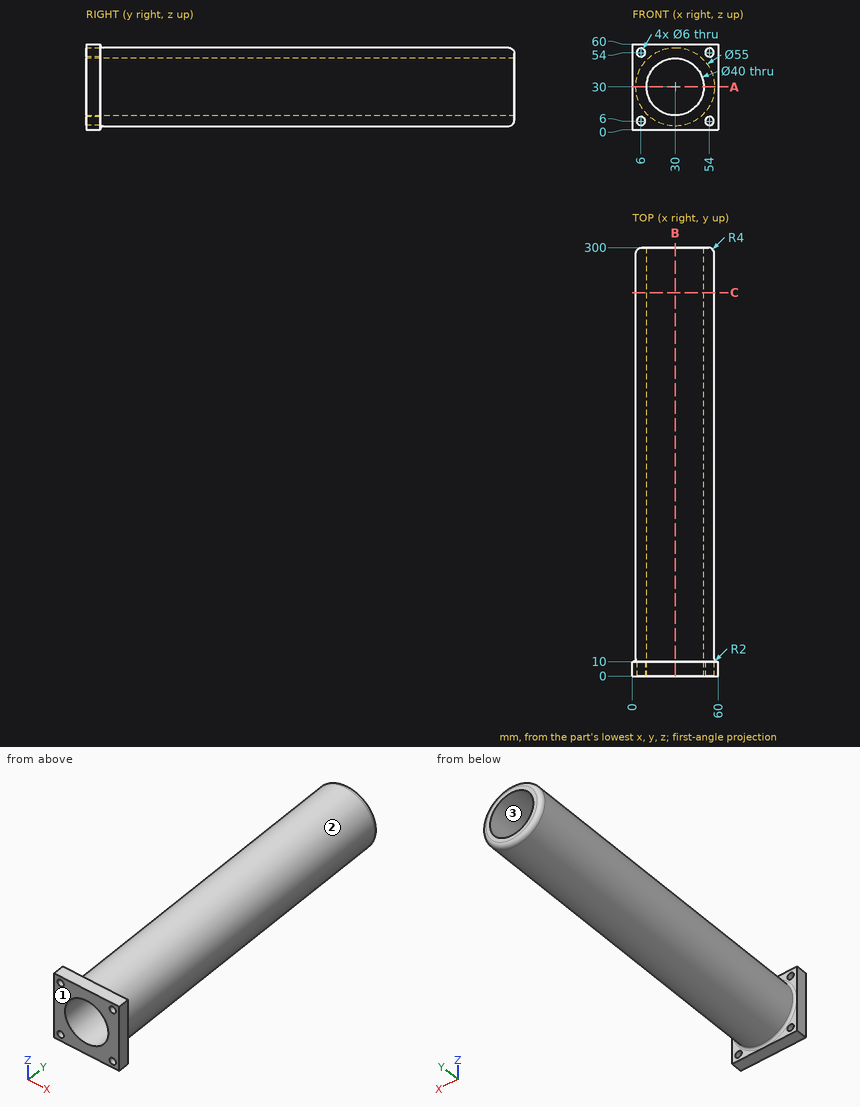
Design review of the part shown in the three views and the two pictorial views. Dimensions are in mm from the part's minimum x, y and z. Give positions to 0.01 mm unless a question says otherwise; leave off trailing zeros. Loops run counter-clockwise (first coordinate to the right, second up) from the corner with the lowest first, then second, coordinate; pieces in that order, holes last. Notation, with made-up numbers: (20, 55.25) -> (77, 55.25) arc R32 cw to (77, 93.25) -> close; hole circle Ø9 at (6.5, -16). An arc over 180 degrees is marked (long way). Write each question's results on one line, items separated by ' | '.
Q1. Wall thickness on L1, parallel to Z at x = 54, y = 4.25; L2, parallel to Z at x = 28.5, y = 36: over which ranges is each line inside the solid? List them lowest first.
Reply:
L1: z = 0 to 3, 9 to 51, 57 to 60 | L2: z = 2.54 to 10.06, 49.94 to 57.46
Q2. Take a section at B-B, the plane x = 30. Write out the cut boundary in (y, z), plus the area to 3 significant figures.
Reply:
outline: (0, 0) -> (10, 0) -> (10, 0.5) arc R2 cw to (12, 2.5) -> (296, 2.5) arc R4 ccw to (300, 6.5) -> (300, 10) -> (0, 10) -> close; (0, 50) -> (300, 50) -> (300, 53.5) arc R4 ccw to (296, 57.5) -> (12, 57.5) arc R2 cw to (10, 59.5) -> (10, 60) -> (0, 60) -> close | area: 4,540 mm²
Q3. For pin 1 Ø3 at (y, z) = (143, 26.5) entering from -X; pin 2 Ø1 at (x, y) = (12.5, 148) entering from -Z; pin 3 Ø3 at (x, y) = (19.5, 105.5) entering from -Z, all flat-tipped, find the tip position at first contact; note any pin that passes through.
Reply:
pin 1: stops at x = 2.57 | pin 2: stops at z = 8.38 | pin 3: stops at z = 4.01
Q4. The part is to be moulded in two halves that separate along Z. For the marked faces 1, 2 and 3, say which applies: +Z half, -Z half, draft (parallel to the pull), parting line (faces both ways), or undercut.
Reply:
face 1: draft | face 2: parting line | face 3: undercut
Q5. Take a section at C-C, the plane y = 268.5. Write out the cut boundary in (x, z).
Reply:
outline: circle Ø55 at (30, 30); hole circle Ø40 at (30, 30)
Q6. Take a section at A-A, the plane z = 30. Write out the cut boundary in (x, y).
Reply:
outline: (0, 0) -> (10, 0) -> (10, 300) -> (6.5, 300) arc R4 ccw to (2.5, 296) -> (2.5, 12) arc R2 cw to (0.5, 10) -> (0, 10) -> close; (50, 0) -> (60, 0) -> (60, 10) -> (59.5, 10) arc R2 cw to (57.5, 12) -> (57.5, 296) arc R4 ccw to (53.5, 300) -> (50, 300) -> close
